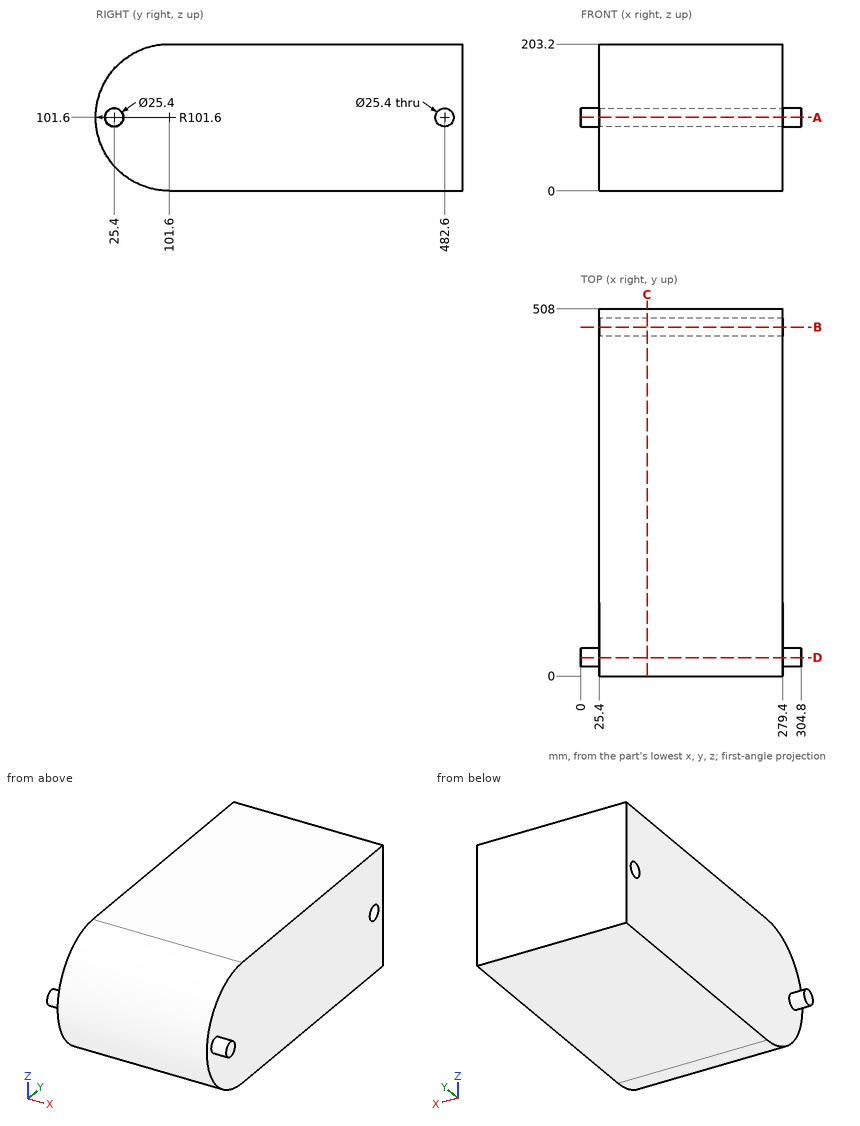
Check sheet for the drawn part. Datum: minimum x, y, z corner. Units: mm. Coordinates: 2 decimals unless noted, no trailing zeros. Loops run counter-clockwise (first coordinate to the right, second up) from the corner with the lowest first, then second, coordinate; pieces in that order, holes last. Notation, with made-up numbers: (62.5, -29.5) -> (84.5, -29.5) arc R5 ccw to (84.5, -21.5) -> close; hole circle Ø1 at (50, 61). An arc over 180 degrees is marked (long way). Answer in a Markdown table with one row per item.
1) Section check C-C (x = 91.5). Record the cut outline in (y, z), and give its area (3 significant figures).
The answers:
| item | result |
|---|---|
| outline | (101.6, 0) -> (508, 0) -> (508, 203.2) -> (101.6, 203.2) arc R101.6 ccw to start; hole circle Ø25.4 at (482.6, 101.6) |
| area | 98,300 mm2 |
2) Section check D-D (y = 25.4). Record the cut outline in (x, z).
The answers:
| item | result |
|---|---|
| outline | (0, 88.9) -> (25.4, 88.9) -> (25.4, 34.4) -> (279.4, 34.4) -> (279.4, 88.9) -> (304.8, 88.9) -> (304.8, 114.3) -> (279.4, 114.3) -> (279.4, 168.8) -> (25.4, 168.8) -> (25.4, 114.3) -> (0, 114.3) -> close |
3) Scan lines: line 1 along Z through (x, y) = (222, 482); line 2 along Y through (x, z) = (178, 101); line 3 along X through (y, z) = (386.5, 126.5). Record each from-to range of solid material in increasing order. Write a range as from..to.
The answers:
| item | result |
|---|---|
| line 1 | z = 0..88.91, 114.29..203.2 |
| line 2 | y = 0..469.91, 495.29..508 |
| line 3 | x = 25.4..279.4 |
4) Section check A-A (z = 101.6). Record the cut outline in (x, y).
The answers:
| item | result |
|---|---|
| outline | (0, 12.7) -> (25.4, 12.7) -> (25.4, 0) -> (279.4, 0) -> (279.4, 12.7) -> (304.8, 12.7) -> (304.8, 38.1) -> (279.4, 38.1) -> (279.4, 469.9) -> (25.4, 469.9) -> (25.4, 38.1) -> (0, 38.1) -> close; (25.4, 495.3) -> (279.4, 495.3) -> (279.4, 508) -> (25.4, 508) -> close |
5) Section check B-B (y = 482.6). Record the cut outline in (x, z).
The answers:
| item | result |
|---|---|
| outline | (25.4, 0) -> (279.4, 0) -> (279.4, 88.9) -> (25.4, 88.9) -> close; (25.4, 114.3) -> (279.4, 114.3) -> (279.4, 203.2) -> (25.4, 203.2) -> close |
6) Depth check by flat-ended pin: P1, Ø12, axis at y = 321, z = 65, coming from the +X side; P2, Ø1.5, axis at y = 454, z = 167, coming from the -X side; P3, Ø12, axis at x = 31, z = 135.5, coming from the -Y side; P4, Ø23, axis at y = 482.6, z = 101.6, coming from the +X side. Enter the tip coordinate at first touch or a pass-through.
The answers:
| item | result |
|---|---|
| P1 | stops at x = 279.4 |
| P2 | stops at x = 25.4 |
| P3 | stops at y = 3.91 |
| P4 | passes through |
